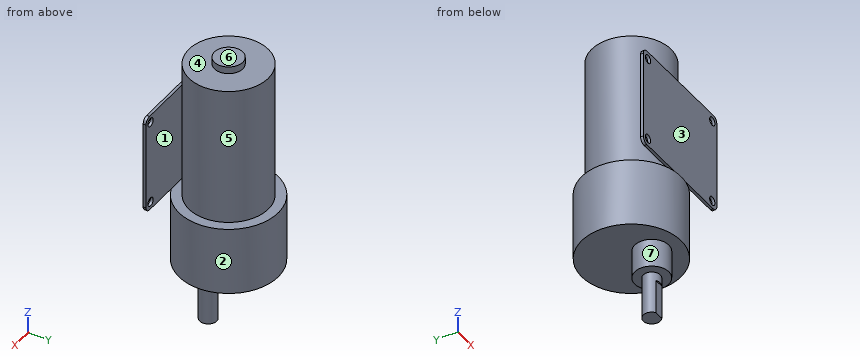
```python
from build123d import *

# Parameters (mm, degrees)
ESQUISSE1_R             = 14
BOSS_EXTRU_1_DEPTH      = 49
ESQUISSE2_R             = 5
BOSS_EXTRU_2_DEPTH      = 2.5
ESQUISSE3_R             = 17.5
BOSS_EXTRU_3_DEPTH      = 24
ESQUISSE4_R             = 6
BOSS_EXTRU_4_DEPTH      = 10
ESQUISSE5_R             = 3
BOSS_EXTRU_5_DEPTH      = 15
ESQUISSE7_OUTSIDE_W     = 59.406
ESQUISSE7_OUTSIDE_H     = 59.406
ENL_V_MAT_EXTRU_1_DEPTH = 12
BOSS_EXTRU_6_DEPTH      = 35
CONG_1_R                = 2
ESQUISSE9_R             = 1.5
ENL_V_MAT_EXTRU_2_DEPTH = 35


with BuildPart() as part:
    # Esquisse1 → Boss.-Extru.1 (new body)
    with BuildSketch(Plane.XY):
        with Locations((9.642437394, 0)):
            Circle(ESQUISSE1_R)
    extrude(amount=BOSS_EXTRU_1_DEPTH)

    # Esquisse2 → Boss.-Extru.2 (add)
    with BuildSketch(Plane.XY.offset(49)):
        with Locations((9.642437394, 0)):
            Circle(ESQUISSE2_R)
    extrude(amount=BOSS_EXTRU_2_DEPTH)

    # Esquisse3 → Boss.-Extru.3 (add)
    with BuildSketch(Plane(origin=(0, 0, 0), x_dir=(-1, 0, 0), z_dir=(0, 0, -1))):
        with Locations((-9.642437394, 0)):
            Circle(ESQUISSE3_R)
    extrude(amount=BOSS_EXTRU_3_DEPTH)

    # Esquisse4 → Boss.-Extru.4 (add)
    with BuildSketch(Plane(origin=(0, 0, -24), x_dir=(-1, 0, 0), z_dir=(0, 0, -1))):
        with Locations((-9.642437394, -7.2)):
            Circle(ESQUISSE4_R)
    extrude(amount=BOSS_EXTRU_4_DEPTH)

    # Esquisse5 → Boss.-Extru.5 (add)
    with BuildSketch(Plane(origin=(0, 0, -34), x_dir=(-1, 0, 0), z_dir=(0, 0, -1))):
        with Locations((-9.642437394, -7.2)):
            Circle(ESQUISSE5_R)
    extrude(amount=BOSS_EXTRU_5_DEPTH)

    # Esquisse7 outside → Enlèv. mat.-Extru.1 (cut)
    with BuildSketch(Plane(origin=(0, 0, -49), x_dir=(-1, 0, 0), z_dir=(0, 0, -1))):
        with Locations((-9.642, 0)):
            Rectangle(ESQUISSE7_OUTSIDE_W, ESQUISSE7_OUTSIDE_H)
        with BuildLine():
            Line((-11.300749789, -9.7), (-7.984124999, -9.7))
            ThreePointArc((-7.984124999, -9.7), (-9.642437394, -4.2), (-11.300749789, -9.7))
        make_face(mode=Mode.SUBTRACT)
    extrude(amount=-ENL_V_MAT_EXTRU_1_DEPTH, mode=Mode.SUBTRACT)

    # Esquisse8 → Boss.-Extru.6 (add)
    with BuildSketch(Plane.XY):
        Polygon((9.642437394, -16.204776279), (30.642437394, -16.204776279), (30.642437394, -17.204776279), (9.642437394, -17.204776279), (-11.357562606, -17.204776279), (-11.357562606, -16.204776279), align=None)
    extrude(amount=BOSS_EXTRU_6_DEPTH)

    # Congé1
    cong_1_edges = [part.edges().sort_by_distance(p)[0] for p in [
        (-11.357562606, -16.704776279, 0),
        (30.642437394, -16.704776279, 0),
        (-11.357562606, -16.704776279, 35),
        (30.642437394, -16.704776279, 35),
    ]]
    fillet(cong_1_edges, radius=CONG_1_R)

    # Esquisse9 → Enlèv. mat.-Extru.2 (cut)
    with BuildSketch(Plane.XZ.offset(17.204776279)):
        with Locations(Location((28.042437394, 32.4, 0), (0, 0, 270))):
            Circle(ESQUISSE9_R)
        with Locations(Location((-8.757562606, 32.4, 0), (0, 0, 270))):
            Circle(ESQUISSE9_R)
        with Locations(Location((-8.757562606, 2.6, 0), (0, 0, 270))):
            Circle(ESQUISSE9_R)
        with Locations(Location((28.042437394, 2.6, 0), (0, 0, 270))):
            Circle(ESQUISSE9_R)
    extrude(amount=-ENL_V_MAT_EXTRU_2_DEPTH, mode=Mode.SUBTRACT)


solid = part.part
```
The model under review builds one solid part; all positions refer to its coordinate system, in mm. Face numbers are marked on the shaded views. A direction names the side the tool comes from. Coordinates: 2 decimals unless noted, no trailing zeros. Write each loop counter-clockwise with the first axis right and the second up, starting at its lowest first coordinate (ties: lowest second). Pieces come first, ordered by that corner, then holes.
1) We need section D-D on z = -2. State the section outline as (x, y) points.
2) We need section C-C on y = 0. State the section outline as (x, z) points.
3) Machinability: for the marked faces 5, 6 and 7, which of the approach directions +Z, -Z, +X, -X, +Y, -Y give a long, thin tool a straight path to every point of the face, cutting with its end or side? Answer none if there is none.
4) We need section A-A on x = -1.5. State the section outline as (y, z) points, then the cut area to 3 significant figures.
5) To check wall thickness, follow probe 1 along X at (y, z) = (-16.5, 2.6); probe 2 along Y at (x, z) = (10, -41); probe 3 along Z at (x, y) = (4, 6.5). State the ranges of each line that lie inside material, in increasing order.
6) We need section B-B on z = 26.5. State the section outline as (x, y) points.
7) Clearance check with flat-ended pins moving along their axes: pin 1 Ø1.5 at (x, y) = (8.5, 8.5) entering from +Z; pin 2 Ø1.7 at (x, z) = (10, -43.5) entering from -Y; pin 3 Ø17.5 at (x, z) = (2.5, 13.5) entering from +Y. State where each tip first meets the part, or that it passes through.
8) The part is to be moulded in two halves that separate along Y. For the marked faces 1, 2, 3 and 4, say which applies: pulls with the +Y half, pulls with the -Y half, needs draft (parallel to the pull), parting line crosses it, or undercut.
Answer list:
1. outline: circle Ø35 at (9.64, 0)
2. outline: (-7.86, -24) - (27.14, -24) - (27.14, 0) - (23.64, 0) - (23.64, 49) - (14.64, 49) - (14.64, 51.5) - (4.64, 51.5) - (4.64, 49) - (-4.36, 49) - (-4.36, 0) - (-7.86, 0) - close
3. face 5: +Z
3. face 6: +Z, +X, -X, +Y, -Y
3. face 7: -Z
4. outline: (-17.2, 0) - (-16.2, 0) - (-16.2, 35) - (-17.2, 35) - close; (-13.49, -24) - (13.49, -24) - (13.49, 0) - (8.48, 0) - (8.48, 49) - (-8.48, 49) - (-8.48, 0) - (-13.49, 0) - close
4. area: 1,510 mm2
5. probe 1: x = -11.36 to -10.26, -7.26 to 26.54, 29.54 to 30.64
5. probe 2: y = -9.7 to -4.22
5. probe 3: z = -24 to 49
6. outline: (-11.36, -17.2) - (30.64, -17.2) - (30.64, -16.2) - (-11.36, -16.2) - close; circle Ø28 at (9.64, 0)
7. pin 1: stops at z = 49
7. pin 2: stops at y = -9.7
7. pin 3: stops at y = 14
8. face 1: undercut
8. face 2: parting line crosses it
8. face 3: pulls with the -Y half
8. face 4: needs draft
